from build123d import *

# Parameters (mm, degrees)
F0_W     = 160
F0_H     = 34
F1_DEPTH = 152.4
F2_R     = 15.773728
F3_DEPTH = 137


with BuildPart() as f1:
    # F0 (on Front) → F1 (new body)
    with BuildSketch(Plane.XZ):
        with Locations((18.404959, 17)):
            Rectangle(F0_W, F0_H)
    extrude(amount=-F1_DEPTH)

    # F2 (on Top) → F3 (join)
    with BuildSketch(Plane.XY):
        with Locations((-36.002856, 24.256775)):
            Circle(F2_R)
    extrude(amount=-F3_DEPTH)


solid = f1.part
For this review, take the finished solid that the model builds, in its own axes (mm). A direction names the side the tool comes from. Coordinates: 2 decimals unless noted, no trailing zeros. Order: outer loops, then holes, each group sorted by start corner. A loop starts at its lowest first (then second) coordinate and runs counter-clockwise, first axis right, second up. Notation, with made-up numbers: (32.5, -11.75) - (66.5, -11.75) arc R22 cw to (66.5, 16.25) - close; hole circle Ø3 at (-18, 47.25). An arc over 180 degrees is marked (long way). Answer as CSV lines item,"result". Start each with the question number.
1) Insertion check: P1, Ø3, axis at x = -25, y = 53.5, coming from the -Z side; P2, Ø12, axis at y = 38, z = -22.5, coming from the -X side; P3, Ø6, axis at x = 14.5, z = 1, coming from the -Y side. Each pin has a flat end and moves straight along its axis. Give the tip position at first contact, or say it passes through.
2) Add section A-A (x = -45). State the section outline as (y, z) points.
3) Add section C-C (z = -75). State the section outline as (x, y) points.
4) Add section B-B (y = 31.5). State the section outline as (x, z) points.
5) Add section D-D (x = -0.5). State the section outline as (y, z) points, then the cut area to 3 significant figures.
6) To check wall thickness, follow line 1 along Z through (x, y) = (87, 42); line 2 along Y through (x, z) = (-42, -107); line 3 along X through (y, z) = (33, -2). State the ranges of each line that lie inside material, in increasing order. Write a range as [from, to].
7) Machinability: for faces 1 (the flat face through (-61.595, 75, 17)), 2 (the cylindrical face through (-20.958, 28.995, -67.541)), which of the approach directions +Z, -Z, +X, -X, +Y, -Y give a long, thin tool a straight path to every point of the face, cutting with its end or side? Answer none if there is none.
Result:
1,P1,"z = 0"
1,P2,"x = -49.75"
1,P3,"y = 0"
2,outline,"(0, 0) - (11.3, 0) - (11.3, -137) - (37.21, -137) - (37.21, 0) - (152.4, 0) - (152.4, 34) - (0, 34) - close"
3,outline,"circle Ø31.55 at (-36, 24.26)"
4,outline,"(-61.6, 0) - (-50.02, 0) - (-50.02, -137) - (-21.99, -137) - (-21.99, 0) - (98.4, 0) - (98.4, 34) - (-61.6, 34) - close"
5,outline,"(0, 0) - (152.4, 0) - (152.4, 34) - (0, 34) - close"
5,area,"5,180 mm^2"
6,line 1,"[0, 34]"
6,line 2,"[9.67, 38.85]"
6,line 3,"[-49.13, -22.87]"
7,face 1,"+Z, -Z, -X, +Y, -Y"
7,face 2,"-Z"
